Could you check a few things on this model? Use its own coordinates, in mm. Face numbers are marked on the shaded views. A direction names the side the tool comes from. Give positions to 0.01 mm unless a question says otherwise; leave off trailing zeros. Loops run counter-clockwise (first coordinate to the right, second up) from the corner with the lowest first, then second, coordinate; pieces in that order, holes last. Notation, with made-up numbers: (-15, -27.75) - (-9, -27.75) arc R22 ccw to (-9, -10.75) - close; hole circle Ø3 at (34.25, 4.5). An arc over 180 degrees is marked (long way). One line per item, written item: value. Start each with the question number.
Q1. If I drill on line 1 (Y direction, x = -67, z = -67); line 2 (Z direction, x = -94.5, y = -29); line 3 (X direction, y = 25.5, z = -15.5), over which ranges is the centre line in solid material (lowest first)? Write a range as from..to.
Q2. If we mould it in two halves opening along Z, with no side actions, what happens to the marked faces 3, 4 and 5? For each: released by +Z, released by -Z, zero draft, split by the parting line, or undercut.
Q3. I'm going to push flat-ended pins straight in: P1, Ø4, axis at x = -41.5, y = 32.5, coming from the -Z side; P2, Ø9.5, axis at x = -128.58, y = 46.18, coming from the -Z side; P3, Ø5, axis at y = -14.5, z = -22.5, coming from the -X side; P4, Ø15, axis at y = 13.5, z = -18, coming from the +X side. Where does each tip first touch, or does it pass through?
Q4. I want a section at D-D (x = -97). Please give me the cut outline in (y, z).
Q5. For the marked faces 1 and 2, which set-ups out of +Z, -Z, +X, -X, +Y, -Y let a thin tool reach every point of the face, with its end or its side?
Q6. I want a section at C-C (y = 43.5). Please give me the cut outline in (x, z), then the cut area to 3 significant figures.
Q7. I want a section at B-B (y = -8). Please give me the cut outline in (x, z).
Q8. I want a section at A-A (x = -80). Please give me the cut outline in (y, z), then the cut area to 3 significant figures.
```python
from build123d import *

# Parameters (mm, degrees)
Y_KSEKLIK_EKSTR_ZYON1_OUTLINE_R = 6
Y_KSEKLIK_EKSTR_ZYON1_DEPTH     = 12
Y_KSEKLIK_EKSTR_ZYON6_DEPTH     = 62


# Read off the part's stored shape, not the designer's step: Yükseklik-Ekstrüzyon1
with BuildPart() as part:
    # Yükseklik-Ekstrüzyon1 outline → Yükseklik-Ekstrüzyon1 (new body)
    with BuildSketch(Plane.XY):
        with BuildLine():
            ThreePointArc((-6.071419214, 35.304785694), (-7.405582554, 59.467641529), (-28.582022208, 71.180113408))
            Line((-28.582022208, 71.180113408), (-128.582022208, 71.180113408))
            ThreePointArc((-128.582022208, 71.180113408), (-149.758461862, 59.467641529), (-151.092625201, 35.304785694))
            Line((-151.092625201, 35.304785694), (-105.594745799, -58.870279849))
            ThreePointArc((-105.594745799, -58.870279849), (-78.582022207, -75.819886592), (-51.569298616, -58.870279849))
            Line((-51.569298616, -58.870279849), (-6.071419214, 35.304785694))
        make_face()
        with Locations((-78.582022208, -45.819886592)):
            Circle(Y_KSEKLIK_EKSTR_ZYON1_OUTLINE_R, mode=Mode.SUBTRACT)
        with Locations((-128.582022208, 46.180113408)):
            Circle(Y_KSEKLIK_EKSTR_ZYON1_OUTLINE_R, mode=Mode.SUBTRACT)
        with Locations((-28.582022208, 46.180113408)):
            Circle(Y_KSEKLIK_EKSTR_ZYON1_OUTLINE_R, mode=Mode.SUBTRACT)
    extrude(amount=Y_KSEKLIK_EKSTR_ZYON1_DEPTH)

    # Çizim6 → Yükseklik-Ekstrüzyon6 (add)
    with BuildSketch(Plane(origin=(0, 46.180113408, 0), x_dir=(1, 0, 0), z_dir=(0, 1, 0))):
        with BuildLine():
            Line((-93.582022208, 0), (-63.582022208, 0))
            Line((-63.582022208, 0), (-63.582022208, 30))
            Line((-63.582022208, 30), (-63.662550873, 30))
            ThreePointArc((-63.662550873, 30), (-78.505910332, 75.116527532), (-93.349269791, 30))
            Line((-93.349269791, 30), (-93.582022208, 30))
            Line((-93.582022208, 30), (-93.582022208, 0))
        make_face()
    extrude(amount=-Y_KSEKLIK_EKSTR_ZYON6_DEPTH)


solid = part.part
```
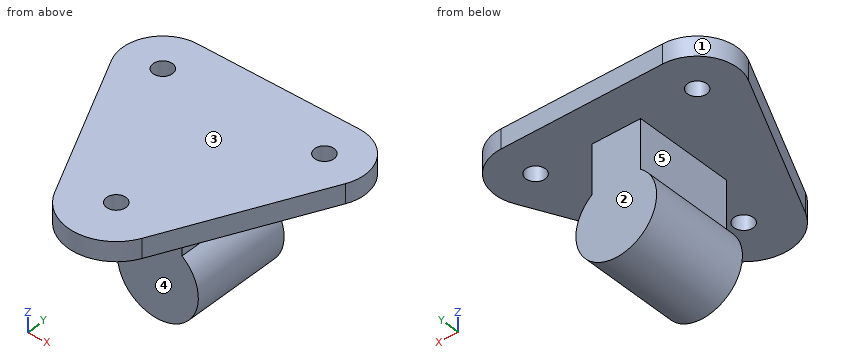
Worked answers:
1. line 1: y = -15.82..46.18
1. line 2: z = 0..12
1. line 3: x = -93.58..-63.58
2. face 3: released by +Z
2. face 4: zero draft
2. face 5: undercut
3. P1: stops at z = 0
3. P2: passes through
3. P3: stops at x = -93.58
3. P4: stops at x = -63.58
4. outline: (-69.5, 0) - (71.18, 0) - (71.18, 12) - (-69.5, 12) - close; (-15.82, -66.94) - (46.18, -66.94) - (46.18, -33.29) - (-15.82, -33.29) - close
5. face 1: +Z, -Z, -X
5. face 2: -Z, +X, -X, +Y
6. outline: (-153.44, 0) - (-133.95, 0) - (-133.95, 12) - (-153.44, 12) - close; (-123.21, 0) - (-93.58, 0) - (-93.58, -30) - (-93.35, -30) arc R25 ccw (long way) to (-63.66, -30) - (-63.58, -30) - (-63.58, 0) - (-33.95, 0) - (-33.95, 12) - (-123.21, 12) - close; (-23.21, 0) - (-3.73, 0) - (-3.73, 12) - (-23.21, 12) - close
6. area: 4,300 mm²
7. outline: (-130.17, 0) - (-93.58, 0) - (-93.58, -30) - (-93.35, -30) arc R25 ccw (long way) to (-63.66, -30) - (-63.58, -30) - (-63.58, 0) - (-26.99, 0) - (-26.99, 12) - (-130.17, 12) - close
8. outline: (-75.79, 0) - (-51.65, 0) - (-51.65, 12) - (-75.79, 12) - close; (-39.99, 0) - (-15.82, 0) - (-15.82, -75.07) - (46.18, -75.07) - (46.18, 0) - (71.18, 0) - (71.18, 12) - (-39.99, 12) - close
8. area: 6,280 mm²
